Read the model definition and answer for the solid it produces. Units are mm, in the model's axes. A direction names the side the tool comes from. Coordinates: 2 decimals unless noted, no trailing zeros. Loops run counter-clockwise (first coordinate to the right, second up) from the corner with the lowest first, then second, coordinate; pieces in that order, holes last.
from build123d import *

# Parameters (mm, degrees)
F0_R     = 38.1
F1_DEPTH = 241.3
F3_D     = 38.1
F3_DEPTH = 50.8
F3_TIP   = 11.4463947925
F5_D     = 38.1
F5_DEPTH = 50.8
F5_TIP   = 11.4463947925


with BuildPart() as f1:
    # F0 (on Right) → F1 (new body, symmetric)
    with BuildSketch(Plane.YZ):
        Circle(F0_R)
    extrude(amount=F1_DEPTH, both=True)

    # F3
    with Locations(Plane(origin=(-241.3, 0, 0), x_dir=(0, -1, 0), z_dir=(-1, 0, 0))):
        with Locations((0, 0)):
            Hole(F3_D / 2, depth=F3_DEPTH)
            with Locations((0, 0, -(F3_DEPTH + F3_TIP / 2))):  # 118° drill point
                Cone(0, F3_D / 2, F3_TIP, mode=Mode.SUBTRACT)

    # F5
    with Locations(Plane.YZ.offset(241.3)):
        with Locations((0, 0)):
            Hole(F5_D / 2, depth=F5_DEPTH)
            with Locations((0, 0, -(F5_DEPTH + F5_TIP / 2))):  # 118° drill point
                Cone(0, F5_D / 2, F5_TIP, mode=Mode.SUBTRACT)


solid = f1.part
Q1. A cutting plane is placed at C-C (y = -31). Give the vertices of the cut face in (x, z), then the cut area to 3 significant figures.
Findings below:
outline: (-241.3, -22.15) - (241.3, -22.15) - (241.3, 22.15) - (-241.3, 22.15) - close
area: 21,400 mm2
Q2. Which of the six approach directions +Z, -Z, +X, -X, +Y, -Y give full straight-line access (tool end or side, diameter ignored) to faces 1 (the face through (215.54, 15.12, -11.59)), 2 (the face through (-215.54, -15.12, -11.59)), 3 (the face through (241.3, 7.9, 17.5))?
Findings below:
face 1: +X
face 2: -X
face 3: +Z, -Z, +X, +Y, -Y
Q3. A cutting plane is placed at A-A (x = 25). Give the vertices of the cut face in (y, z).
Findings below:
outline: circle Ø76.2 at (0, 0)
Q4. Flat-ended cylindrical pins translate along their axes: pin 1 Ø1.5 at (x, z) = (67, 12.5) entering from -Y; pin 2 Ø5 at (x, y) = (82.5, -11) entering from -Z; pin 3 Ø8 at (x, y) = (183, -26) entering from +Z. Find the tip coordinate at first contact, or state that the pin passes through.
Findings below:
pin 1: stops at y = -36.24
pin 2: stops at z = -37.14
pin 3: stops at z = 31.11
Q5. Straight lines are drawn through the part: probe 1 along Z at (x, y) = (-218, 0); probe 2 along Y at (x, z) = (-201.5, -3); probe 3 along Z at (x, y) = (-200, 7.5). For each, find the intervals that lie inside material, in ascending order.
Findings below:
probe 1: z = -38.1 to -19.05, 19.05 to 38.1
probe 2: y = -37.98 to -18.81, 18.81 to 37.98
probe 3: z = -37.35 to -17.51, 17.51 to 37.35
Q6. Determine the mould class of faces 4 (the face through (-181.041, 2.438, 2.236)), 5 (the face through (3.378, -30.235, -23.183)), 6 (the face through (-241.3, 7.9, 17.5)) for opening direction Y: +Y half, -Y half, draft (parallel to the pull), parting line (faces both ways), or undercut.
Findings below:
face 4: undercut
face 5: parting line
face 6: draft
Q7. A cutting plane is placed at B-B (z = -26). Give the vertices of the cut face in (x, y), then the cut area to 3 significant figures.
Findings below:
outline: (-241.3, -27.85) - (241.3, -27.85) - (241.3, 27.85) - (-241.3, 27.85) - close
area: 26,900 mm2
